Part model, mm, in its own coordinate system. A direction names the side the tool comes from. Coordinates: 2 decimals unless noted, no trailing zeros. Write each loop counter-clockwise with the first axis right and the second up, starting at its lowest first coordinate (ties: lowest second). Pieces come first, ordered by that corner, then holes. Notation, with made-up numbers: (28.5, 29.25) -> (52.5, 29.25) arc R20 ccw to (52.5, 56.25) -> close; hole circle Ø11 at (-25.5, 41). An arc over 180 degrees is marked (long way). Write item = value, one per line.
from build123d import *

# Parameters (mm, degrees)
SWEEP1_PROFILE_R   = 30
SKETCH32_R         = 25
CUT_EXTRUDE1_DEPTH = 310
FILLET1_R          = 4


with BuildPart() as part:
    # Sketch1 → Revolve1 (revolve)
    with BuildSketch(Plane(origin=(0, 0, 0), x_dir=(1, 0, 0), z_dir=(0, 1, 0))):
        with BuildLine():
            Line((0, 474.99999), (20, 474.99999))
            Line((20, 474.99999), (20, 0))
            Line((20, 0), (50, 0))
            Line((50, 0), (50, 475))
            ThreePointArc((50, 475), (42.67766953, 492.67766953), (25, 500))
            Line((25, 500), (0, 500))
            Line((0, 500), (0, 474.99999))
        make_face()
    revolve(axis=Axis((0, 0, 0), (0, 0, -1)))

    # Sweep1: sweep along a curve in space
    with BuildLine() as sweep1_path:
        ThreePointArc((0, 0, -312.675247361), (157.645703228, 0, -337.320292822), (300, 0, -265.245330439))
    # Sweep1 profile (on start of the path) → Sweep1 (sweep)
    with BuildSketch(Plane(origin=(0, 0, -312.675247361), x_dir=(0.45016951101566693, 0, 0.892943117646312), z_dir=(0.892943117646312, 0, -0.45016951101566693))):
        Circle(SWEEP1_PROFILE_R)
    sweep(path=sweep1_path.line)

    # Sketch32 → Cut-Extrude1 (cut)
    with BuildSketch(Plane.XY):
        with Locations((230, 0)):
            Circle(SKETCH32_R)
    extrude(amount=-CUT_EXTRUDE1_DEPTH, mode=Mode.SUBTRACT)

    # Fillet1
    fillet1_edges = [part.edges().sort_by_distance(p)[0] for p in [
        (321.110299285, 0, -286.560941247),
    ]]
    fillet(fillet1_edges, radius=FILLET1_R)


solid = part.part
Q1. Probe line 1 (X direction, y = 0, z = -285); line 2 (X direction, y = 0, z = -97.5); line 3 (X direction, y = -1.5, z = -415.5). List the from-to ranges inside material, lowest first. Write a range as from..to.
Model answer:
line_1 = -50..-20, 20..50, 255..319.14
line_2 = -50..-20, 20..50
line_3 = -49.98..-19.94, 19.94..49.98
Q2. Which spindle directions (+Z, -Z, +X, -X, +Y, -Y) get a long thin tool onto all of the face, cutting with end or side? Do faces 1 (the face through (0, 0, -500)), 2 (the face through (253.846, 7.509, -297.055)), 3 (the face through (-19.98, -0.88, -234.17)). Say none if no direction does.
Model answer:
face_1 = -Z, +X, -X, +Y, -Y
face_2 = +Z
face_3 = none
Q3. Saw through at A-A on z = -98. Give the cut face in (x, y), and give its area (3 significant figures).
Model answer:
outline = circle Ø100 at (0, 0); hole circle Ø40 at (0, 0)
area = 6,600 mm²
Q4. Mould opens along X. For faces 4 (the face through (-0.19, -0.28, -313.05)), 5 (the face through (300.23, -0.41, -265.48)), 6 (the face through (230, 0, -310)), 7 (the face through (1, 22, 0)) say: released by +X, released by -X, zero draft, split by the parting line, or undercut.
Model answer:
face_4 = undercut
face_5 = released by +X
face_6 = undercut
face_7 = zero draft
Q5. Pin check, flat tips, straight feed: pin 1 (8 mm diameter, centred on x = 172, y = 27, fed in from +Z); pin 2 (5 mm diameter, centred on y = 20.5, z = -59.5, fed in from -X); pin 3 (20 mm diameter, centred on x = 8.5, y = 3.5, fed in from +Z). Stop position of each tip, or through.
Model answer:
pin_1 = -314.8
pin_2 = -46.65
pin_3 = -285.89
